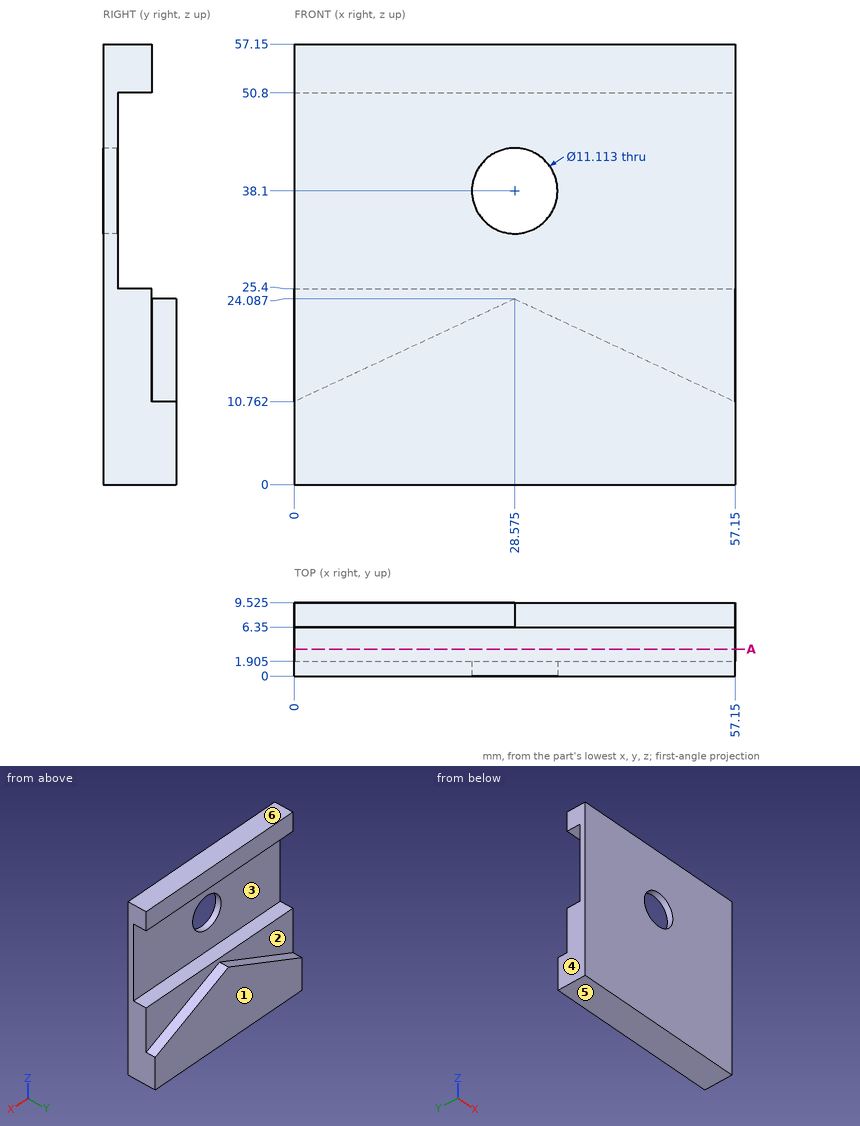
Can you work these out from the drawing? Everything is in mm from the part's minimum corner. A direction names the side the tool comes from. Round coordinates to 2 decimals unless told otherwise and drop trailing zeros. Loops run counter-clockwise (first coordinate to the right, second up) from the corner with the lowest first, then second, coordinate; pieces in that order, holes last. Notation, with made-up numbers: (-22, 35.25) - (6, 35.25) arc R13 cw to (6, 44.25) - close; hole circle Ø11 at (-18, 50). An arc over 180 degrees is marked (long way). Answer as CSV lines item,"result".
1. Please list where these lines run through material, in increasing order: line 1 along Z through (x, y) = (28, 4); line 2 along X through (y, z) = (0.7, 38.1); line 3 along Y through (x, z) = (44, 40) (1 decimal). Write a range as [from, to].
Filled in:
line 1,"z = [0, 25.4], [50.8, 57.15]"
line 2,"x = [0, 23.02], [34.13, 57.15]"
line 3,"y = [0, 1.9]"
2. For pin 1 Ø1.5 at (x, z) = (9.5, 5.5) entering from -Y; pin 2 Ø5 at (x, z) = (48.5, 45) entering from +Y (1 decimal); pin 3 Ø5 at (x, z) = (20, 53.5) entering from +Y, each with a flat end and sliding along its axis, tell me the tip position at first contact or that it passes through.
Filled in:
pin 1,"stops at y = 0"
pin 2,"stops at y = 1.9"
pin 3,"stops at y = 6.35"
3. On a 3-axis mill with a long thin cutter (end or side, diameter ignored), from which of +Z, -Z, +X, -X, +Y, -Y can I reach the whole of each face in a straight line? I mean the marked faces 1 and 2. Say none if no direction works.
Filled in:
face 1,"+Z, -Z, +X, -X, +Y"
face 2,"+Z, +Y"
4. I want a section at A-A on y = 3.5. List the corners of the cut face in (x, z) for me, then the cut area to 3 significant figures.
Filled in:
outline,"(0, 0) - (57.15, 0) - (57.15, 25.4) - (0, 25.4) - close; (0, 50.8) - (57.15, 50.8) - (57.15, 57.15) - (0, 57.15) - close"
area,"1,810 mm^2"
5. We'd pull the mould along Z, two halves only. Please class the marked faces 3, 4, 5 and 6: +Z half, -Z half, draft (parallel to the pull), parting line (faces both ways), or undercut.
Filled in:
face 3,"undercut"
face 4,"draft"
face 5,"-Z half"
face 6,"+Z half"
